Source: CAD feature listing. Evaluate the final solid. Frame: model axes, mm. A direction names the side the tool comes from. Give positions to 0.01 mm unless a question says otherwise; leave off trailing zeros. Loops run counter-clockwise (first coordinate to the right, second up) from the corner with the lowest first, then second, coordinate; pieces in that order, holes last. Notation, with made-up numbers: M -22.5,63.5 L -6.5,63.5 A28 cw -6.5,85.5 Z; hole C 69.25,-14 d1. An arc over 180 degrees is marked long. Answer in a Markdown table with one row per item.
```python
from build123d import *

# Parameters (mm, degrees)
SKETCH1_W           = 50
SKETCH1_H           = 30
BOSS_EXTRUDE1_DEPTH = 5
SKETCH2_W           = 4
SKETCH2_H           = 1
CUT_EXTRUDE1_DEPTH  = 2
SKETCH3_R           = 4.5
CUT_EXTRUDE2_DEPTH  = 22
SKETCH3_3_R         = 4.5
SKETCH3_3_R_2       = 1.5
CUT_EXTRUDE3_DEPTH  = 22
CHAMFER1_SIZE       = 1


with BuildPart() as part:
    # Sketch1 → Boss-Extrude1 (new body)
    with BuildSketch(Plane(origin=(0, 0, 0), x_dir=(1, 0, 0), z_dir=(0, 1, 0))):
        Rectangle(SKETCH1_W, SKETCH1_H)
    extrude(amount=BOSS_EXTRUDE1_DEPTH)

    # Sketch2 → Cut-Extrude1 (cut)
    with BuildSketch(Plane(origin=(0, 5, 0), x_dir=(1, 0, 0), z_dir=(0, 1, 0))):
        with Locations((23, 0)):
            Rectangle(SKETCH2_W, SKETCH2_H)
    extrude(amount=-CUT_EXTRUDE1_DEPTH, mode=Mode.SUBTRACT)

    # Sketch3 → Cut-Extrude2 (cut)
    with BuildSketch(Plane(origin=(0, 5, 0), x_dir=(1, 0, 0), z_dir=(0, 1, 0))):
        with Locations((5.4, 0)):
            Circle(SKETCH3_R)
    extrude(amount=-CUT_EXTRUDE2_DEPTH, mode=Mode.SUBTRACT)

    # Sketch3<3> → Cut-Extrude3 (cut)
    with BuildSketch(Plane(origin=(0, 5, 0), x_dir=(1, 0, 0), z_dir=(0, 1, 0))):
        with Locations((5.4, 0)):
            Circle(SKETCH3_3_R)
        with Locations((-21, 11)):
            Circle(SKETCH3_3_R_2)
        with Locations((21, 11)):
            Circle(SKETCH3_3_R_2)
        with Locations((21, -11)):
            Circle(SKETCH3_3_R_2)
        with Locations((-21, -11)):
            Circle(SKETCH3_3_R_2)
    extrude(amount=-CUT_EXTRUDE3_DEPTH, mode=Mode.SUBTRACT)

    # Chamfer1
    chamfer1_edges = [part.edges().sort_by_distance(p)[0] for p in [
        (0, 0, 15),
        (-25, 0, 0),
        (0, 0, -15),
        (25, 0, 0),
        (25, 2.5, 15),
        (-25, 2.5, 15),
        (-25, 2.5, -15),
        (25, 2.5, -15),
    ]]
    chamfer(chamfer1_edges, length=CHAMFER1_SIZE)


solid = part.part
```
Q1. Section query B-B (z = -11). Output: boundary loops of the cut face in (x, y).
Values follow:
| item | result |
|---|---|
| outline | M -25,1 L -24,0 L -22.5,0 L -22.5,5 L -25,5 Z; M -19.5,0 L 19.5,0 L 19.5,5 L -19.5,5 Z; M 22.5,0 L 24,0 L 25,1 L 25,5 L 22.5,5 Z |
Q2. Contact query for a flat-ended pin moving along its axis: pin 1 Ø0.8 at (y, z) = (3.5, 0) entering from +X. Output: stop coordinate, or through.
Values follow:
| item | result |
|---|---|
| pin 1 | x = 21 |
Q3. Reachability of faces 1 (the flat face through (24.5, 3, -14.5)), 2 (the flat face through (23, 3, 0)) from +Z, -Z, +X, -X, +Y, -Y: full face, straight path, thin tool, end or side. Return the list, or none.
Values follow:
| item | result |
|---|---|
| face 1 | -Z, +X, +Y, -Y |
| face 2 | +X, +Y |
Q4. Mould query, pull axis Z, two halves, no side actions, for faces 3 (the flat face through (21, 4, 0)), 4 (the flat face through (-24.3, 0.7, -14.4)), 5 (the flat face through (-24.4, 0.7, 14.3)). Classes: +Z half, -Z half, draft (parallel to the pull), parting line (faces both ways), or undercut.
Values follow:
| item | result |
|---|---|
| face 3 | undercut |
| face 4 | -Z half |
| face 5 | +Z half |
Q5. Section query A-A (x = -21). Output: boundary loops of the cut face in (y, z).
Values follow:
| item | result |
|---|---|
| outline | M 0,-14 L 1,-15 L 5,-15 L 5,-12.5 L 0,-12.5 Z; M 0,-9.5 L 5,-9.5 L 5,9.5 L 0,9.5 Z; M 0,12.5 L 5,12.5 L 5,15 L 1,15 L 0,14 Z |
Q6. Section query C-C (z = 0). Output: boundary loops of the cut face in (x, y), plus the area to 3 significant figures.
Values follow:
| item | result |
|---|---|
| outline | M -25,1 L -24,0 L 0.9,0 L 0.9,5 L -25,5 Z; M 9.9,0 L 24,0 L 25,1 L 25,3 L 21,3 L 21,5 L 9.9,5 Z |
| area | 196 mm^2 |
Q7. Ray query, probe 1 along Z at (x, y) = (-21, 1.5); probe 2 along Z at (x, y) = (5.4, 3.65); probe 3 along X at (y, z) = (3.55, -11). Return the intervals inside material, ascending. Write a range as from..to.
Values follow:
| item | result |
|---|---|
| probe 1 | -15..-12.5, -9.5..9.5, 12.5..15 |
| probe 2 | -15..-4.5, 4.5..15 |
| probe 3 | -25..-22.5, -19.5..19.5, 22.5..25 |
Q8. Section query D-D (y = 1.8). Output: boundary loops of the cut face in (x, z).
Values follow:
| item | result |
|---|---|
| outline | M -25,-14 L -24,-15 L 24,-15 L 25,-14 L 25,14 L 24,15 L -24,15 L -25,14 Z; hole C -21,-11 d3; hole C -21,11 d3; hole C 5.4,0 d9; hole C 21,-11 d3; hole C 21,11 d3 |
